Geometry check sheet. Reference: the model listing, model coordinates, mm. Round coordinates to 2 decimals unless told otherwise and drop trailing zeros. Order: outer loops, then holes, each group sorted by start corner. A loop starts at its lowest first (then second) coordinate and runs counter-clockwise, first axis right, second up. Notation, with made-up numbers: (88, 24) - (142, 24) arc R18 ccw to (142, 48) - close; hole circle Ø1 at (-16, 13.5). An arc over 180 degrees is marked (long way). Answer as CSV lines item,"result". Start each with the question number.
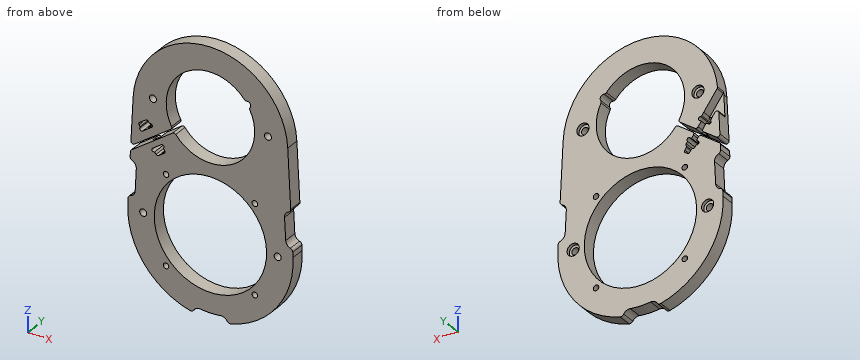
```python
from build123d import *

# Parameters (mm, degrees)
SKETCH1_R           = 40
SKETCH1_R_2         = 50.8
SKETCH1_R_3         = 2.5
BOSS_EXTRUDE1_DEPTH = 12.7
CUT_EXTRUDE1_DEPTH  = 194.127134292
CUT_EXTRUDE2_DEPTH  = 8.5
CUT_EXTRUDE3_DEPTH  = 8.5
CUT_EXTRUDE4_DEPTH  = 194.127134292
CUT_EXTRUDE5_DEPTH  = 8.5
FILLET1_R           = 2
FILLET2_R           = 2
FILLET3_R           = 1.6
FILLET4_R           = 1
SKETCH10_R          = 3.175
CUT_EXTRUDE6_DEPTH  = 194.127134292
SKETCH11_R          = 3
CUT_EXTRUDE7_DEPTH  = 194.127134292
FILLET5_R           = 2
SKETCH12_R          = 5.5
CUT_EXTRUDE8_DEPTH  = 3
CUT_EXTRUDE9_DEPTH  = 194.12713443
FILLET6_R           = 3


with BuildPart() as part:
    # Sketch1 → Boss-Extrude1 (new body)
    with BuildSketch(Plane(origin=(0, 0, 0), x_dir=(1, 0, 0), z_dir=(0, 1, 0))):
        with BuildLine():
            Line((-74.704056398, 99.012658228), (-69.910213207, 4.455696203))
            ThreePointArc((-69.910213207, 4.455696203), (0, -62), (69.910213207, 4.455696203))
            Line((69.910213207, 4.455696203), (74.704056398, 99.012658228))
            ThreePointArc((74.704056398, 99.012658228), (0, 177.6), (-74.704056398, 99.012658228))
        make_face()
        with Locations(Location((0, 0, 0), (0, 0, 270))):
            Circle(SKETCH1_R, mode=Mode.SUBTRACT)
        with Locations(Location((0, 102.8, 0), (0, 0, 270))):
            Circle(SKETCH1_R_2, mode=Mode.SUBTRACT)
        with Locations(Location((40.163665171, 142.963665171, 0), (0, 0, 270))):
            Circle(SKETCH1_R_3, mode=Mode.SUBTRACT)
        with Locations(Location((40.163665171, 62.636334829, 0), (0, 0, 270))):
            Circle(SKETCH1_R_3, mode=Mode.SUBTRACT)
        with Locations(Location((-40.163665171, 62.636334829, 0), (0, 0, 270))):
            Circle(SKETCH1_R_3, mode=Mode.SUBTRACT)
        with Locations(Location((-40.163665171, 142.963665171, 0), (0, 0, 270))):
            Circle(SKETCH1_R_3, mode=Mode.SUBTRACT)
    extrude(amount=BOSS_EXTRUDE1_DEPTH)

    # Sketch3 → Cut-Extrude1 (cut, through all)
    with BuildSketch(Plane(origin=(0, 12.7, 0), x_dir=(1, 0, 0), z_dir=(0, 1, 0))):
        Polygon((0, 0), (-72.307134802, 51.734177215), (-74.169151375, 49.131698727), (-1.862016573, -2.602478489), align=None)
    extrude(amount=-CUT_EXTRUDE1_DEPTH, mode=Mode.SUBTRACT)

    # Sketch4 → Cut-Extrude2 (cut)
    with BuildSketch(Plane(origin=(0, 12.7, 0), x_dir=(1, 0, 0), z_dir=(0, 1, 0))):
        Polygon((-55.43094311, 35.72491958), (-72.445263355, 11.944571389), (-69.985011402, 5.93106572), (-50.957933208, 32.524578595), align=None)
    extrude(amount=-CUT_EXTRUDE2_DEPTH, mode=Mode.SUBTRACT)

    # Sketch5 → Cut-Extrude3 (cut)
    with BuildSketch(Plane(origin=(0, 12.7, 0), x_dir=(1, 0, 0), z_dir=(0, 1, 0))):
        Polygon((-50.957933208, 32.524578595), (-39.203953593, 48.952724054), (-43.676963495, 52.153065038), (-55.43094311, 35.72491958), align=None)
    extrude(amount=-CUT_EXTRUDE3_DEPTH, mode=Mode.SUBTRACT)

    # Sketch6 → Cut-Extrude4 (cut, through all)
    with BuildSketch(Plane(origin=(0, 12.7, 0), x_dir=(1, 0, 0), z_dir=(0, 1, 0))):
        with BuildLine():
            Line((-61.399034012, 31.387778703), (-53.136164811, 25.475876085))
            ThreePointArc((-53.136164811, 25.475876085), (-52.765933853, 23.243628554), (-54.998181384, 22.873397596))
            Line((-54.998181384, 22.873397596), (-57.209326064, 19.782954391))
            Line((-57.209326064, 19.782954391), (-65.472195265, 25.694857009))
            Line((-65.472195265, 25.694857009), (-63.261050585, 28.785300214))
            ThreePointArc((-63.261050585, 28.785300214), (-63.631281543, 31.017547745), (-61.399034012, 31.387778703))
        make_face()
        with BuildLine():
            Line((-48.253577172, 49.279546767), (-40.446141706, 43.693497049))
            Line((-40.446141706, 43.693497049), (-42.657286386, 40.603053844))
            ThreePointArc((-42.657286386, 40.603053844), (-42.287055428, 38.370806313), (-44.519302959, 38.000575355))
            Line((-44.519302959, 38.000575355), (-52.326738425, 43.586625073))
            ThreePointArc((-52.326738425, 43.586625073), (-52.696969382, 45.818872604), (-50.464721852, 46.189103562))
            Line((-50.464721852, 46.189103562), (-48.253577172, 49.279546767))
        make_face()
    extrude(amount=-CUT_EXTRUDE4_DEPTH, mode=Mode.SUBTRACT)

    # Sketch7 → Cut-Extrude5 (cut)
    with BuildSketch(Plane(origin=(0, 12.7, 0), x_dir=(1, 0, 0), z_dir=(0, 1, 0))):
        Polygon((-57.209326064, 19.782954391), (-69.762440014, 2.237885514), (-73.208758404, 10.192307077), (-70.622080139, 18.497034605), (-65.472195265, 25.694857009), align=None)
    extrude(amount=-CUT_EXTRUDE5_DEPTH, mode=Mode.SUBTRACT)

    # Fillet1
    fillet1_edges = [part.edges().sort_by_distance(p)[0] for p in [
        (-32.530981106, 6.35, -23.275207158),
        (-34.288731446, 6.35, -20.598128455),
        (-72.100144873, 6.35, -47.65136972),
        (-72.307134802, 6.35, -51.734177215),
    ]]
    fillet(fillet1_edges, radius=FILLET1_R)

    # Fillet2
    fillet2_edges = [part.edges().sort_by_distance(p)[0] for p in [
        (-70.622080139, 8.45, -18.497034605),
        (-69.762440014, 8.45, -2.237885514),
        (-55.43094311, 8.45, -35.72491958),
        (-50.957933208, 8.45, -32.524578595),
        (-53.568926538, 8.45, -38.327398068),
        (-49.095916635, 8.45, -35.127057084),
    ]]
    fillet(fillet2_edges, radius=FILLET2_R)

    # Fillet3
    fillet3_edges = [part.edges().sort_by_distance(p)[0] for p in [
        (-57.209326064, 2.1, -19.782954391),
        (-65.472195265, 2.1, -25.694857009),
        (-48.253577172, 6.35, -49.279546767),
        (-40.446141706, 6.35, -43.693497049),
        (-39.203953593, 8.45, -48.952724054),
        (-43.676963495, 8.45, -52.153065038),
    ]]
    fillet(fillet3_edges, radius=FILLET3_R)

    # Fillet4
    # the kernel refuses this fillet: 1 mm, written as the material it takes off along each edge
    with BuildSketch(Plane(origin=(-54.998181384, 14.7, -22.873397596), x_dir=(0.9115973776641382, 0, 0.41108420188066924), z_dir=(0, -1, 0))) as fillet4_piece_1:
        with BuildLine():
            CenterArc((0.823687768, 0.980580676), FILLET4_R, 191.309932474, 67.380135052)
            Line((-0.156892908, 0.784464541), (0, 0))
            ThreePointArc((0, 0), (0.313785816, 0.031070919), (0.627571632, 0))
        make_face()
    extrude(amount=16.7, mode=Mode.SUBTRACT)
    with BuildSketch(Plane(origin=(-63.261050585, 14.7, -28.785300214), x_dir=(-0.6833651940435568, 0, -0.7300767162222146), z_dir=(0, -1, 0))) as fillet4_piece_2:
        with BuildLine():
            CenterArc((0.823687768, -0.980580676), FILLET4_R, 101.309932474, 67.380135052)
            Line((-0.156892908, -0.784464541), (0, 0))
            ThreePointArc((0, 0), (0.313785816, -0.031070919), (0.627571632, 0))
        make_face()
    extrude(amount=16.7, mode=Mode.SUBTRACT)
    with BuildSketch(Plane(origin=(-42.113354488, 15.05290288, -44.886351416), x_dir=(0.5818801789556023, 0, -0.8132745276587705), z_dir=(0, -1, 0)), Plane(origin=(-46.58636439, 4.2, -48.0866924), x_dir=(0.5818801789556058, 0, -0.813274527658768), z_dir=(0, 1, 0))) as fillet4_piece_3:
        with BuildLine():
            CenterArc((0.941161152, 1), FILLET4_R, 192.212525269, 77.787474731)
            Line((-0.036208522, 0.788461538), (-0.133945489, 0.767307692))
            ThreePointArc((-0.133945489, 0.767307692), (-0.1, 0.45), (-0.1, 0))
            Line((-0.1, 0), (0, -0.1))
            Line((0, -0.1), (0.941161152, -0.1))
            Line((0.941161152, -0.1), (0.941161152, 0))
        make_face()
    extrude(amount=10.85290288, mode=Mode.SUBTRACT)

    # Sketch10 → Cut-Extrude6 (cut, through all)
    with BuildSketch(Plane(origin=(0, 12.7, 0), x_dir=(1, 0, 0), z_dir=(0, 1, 0))):
        with Locations(Location((-52, 0, 0), (0, 0, 270))):
            Circle(SKETCH10_R)
        with Locations(Location((-60.8, 102.8, 0), (0, 0, 270))):
            Circle(SKETCH10_R)
        with Locations(Location((60.8, 102.8, 0), (0, 0, 90))):
            Circle(SKETCH10_R)
        with Locations(Location((52, 0, 0), (0, 0, 90))):
            Circle(SKETCH10_R)
    extrude(amount=-CUT_EXTRUDE6_DEPTH, mode=Mode.SUBTRACT)

    # Sketch11 → Cut-Extrude7 (cut, through all)
    with BuildSketch(Plane(origin=(0, 12.7, 0), x_dir=(1, 0, 0), z_dir=(0, 1, 0))):
        with Locations((33.397146804, -22.01432682)):
            Circle(SKETCH11_R)
    extrude(amount=-CUT_EXTRUDE7_DEPTH, mode=Mode.SUBTRACT)

    # Fillet5
    fillet5_edges = [part.edges().sort_by_distance(p)[0] for p in [
        (34.95313052, 6.35, 19.449387313),
        (31.653304138, 6.35, 24.455435739),
    ]]
    fillet(fillet5_edges, radius=FILLET5_R)

    # Sketch12 → Cut-Extrude8 (cut)
    with BuildSketch(Plane(origin=(0, 12.7, 0), x_dir=(1, 0, 0), z_dir=(0, 1, 0))):
        with Locations(Location((-60.8, 102.8, 0), (0, 0, 270))):
            Circle(SKETCH12_R)
        with Locations(Location((60.8, 102.8, 0), (0, 0, 270))):
            Circle(SKETCH12_R)
        with Locations(Location((52, 0, 0), (0, 0, 270))):
            Circle(SKETCH12_R)
        with Locations(Location((-52, 0, 0), (0, 0, 270))):
            Circle(SKETCH12_R)
    extrude(amount=-CUT_EXTRUDE8_DEPTH, mode=Mode.SUBTRACT)

    # Sketch13 → Cut-Extrude9 (cut, through all)
    with BuildSketch(Plane(origin=(0, 12.7, 0), x_dir=(1, 0, 0), z_dir=(0, 1, 0))):
        with BuildLine():
            Line((-67.031392983, 66.171925083), (-68.044051211, 86.146271714))
            ThreePointArc((-68.044051211, 86.146271714), (-74.340152668, 91.834778235), (-80.028659189, 85.538676777))
            Line((-80.028659189, 85.538676777), (-79.016000961, 65.564330147))
            ThreePointArc((-79.016000961, 65.564330147), (-72.719899504, 59.875823626), (-67.031392983, 66.171925083))
        make_face()
        with BuildLine():
            Line((67.031392983, 66.171925083), (68.044051211, 86.146271714))
            ThreePointArc((68.044051211, 86.146271714), (74.340152668, 91.834778235), (80.028659189, 85.538676777))
            Line((80.028659189, 85.538676777), (79.016000961, 65.564330147))
            ThreePointArc((79.016000961, 65.564330147), (72.719899504, 59.875823626), (67.031392983, 66.171925083))
        make_face()
        with BuildLine():
            ThreePointArc((10.777978726, 182.877931883), (0, 183.6), (-10.777978726, 182.877931883))
            ThreePointArc((-10.777978726, 182.877931883), (-15.924014851, 176.131205847), (-9.177288816, 170.985169722))
            ThreePointArc((-9.177288816, 170.985169722), (0, 171.6), (9.177288816, 170.985169722))
            ThreePointArc((9.177288816, 170.985169722), (15.924014851, 176.131205847), (10.777978726, 182.877931883))
        make_face()
    extrude(amount=-CUT_EXTRUDE9_DEPTH, mode=Mode.SUBTRACT)

    # Fillet6
    fillet6_edges = [part.edges().sort_by_distance(p)[0] for p in [
        (-74.340152668, 6.35, -91.834778235),
        (-72.719899504, 6.35, -59.875823626),
        (74.340152668, 6.35, -91.834778235),
        (72.719899504, 6.35, -59.875823626),
        (-15.887130952, 6.35, -175.893358591),
        (15.887130952, 6.35, -175.893358591),
    ]]
    fillet(fillet6_edges, radius=FILLET6_R)


solid = part.part
```
1. Thickness scan on probe 1 along X at (y, z) = (10.4, -102.8); probe 2 along Z at (x, y) = (-35.5, 7.5); probe 3 along Z at (x, y) = (33, 8.5). Record the ranges inside material, lowest first.
2. Section check C-C on x = 60.8. Record the boundary of the cut face in (y, z) (3 decimals).
3. Section check A-A on x = 0. Record the boundary of the cut face in (y, z), plus the area to 3 significant figures.
4. Section check B-B on z = -102.8. Record the boundary of the cut face in (x, y) (3 decimals), plus the area to 3 significant figures.
5. Go/stop test with flat-tipped pins: pin 1 Ø5.5 at (x, z) = (62.5, -103) entering from +Y; pin 2 Ø1 at (x, y) = (44.5, 11) entering from -Z; pin 3 Ø3 at (x, y) = (-28, 3.5) entering from -Z. Record where each tip stops, or that it passes through.
6. Section check D-D on y = 7.5. Count the separate pieces of the cut face and the enclosed holes in it, plus the area to 3 significant figures.
Numbers:
1,probe 1,"x = -74.8 to -66.3, -55.3 to -50.8, 50.8 to 55.3, 66.3 to 74.8"
1,probe 2,"z = -168.64 to -139.14, -66.46 to -25.4, -21.43 to -18.43, 18.43 to 52.33"
1,probe 3,"z = -169.93 to -141.42, -64.18 to -22.61, 24.99 to 53.73"
2,outline,"(0, -146.371) - (12.7, -146.371) - (12.7, -108.3) - (9.7, -108.3) - (9.7, -105.975) - (0, -105.975) - close; (0, -99.625) - (9.7, -99.625) - (9.7, -97.3) - (12.7, -97.3) - (12.7, 26.689) - (0, 26.689) - close"
3,outline,"(0, -171.6) - (12.7, -171.6) - (12.7, -153.6) - (0, -153.6) - close; (0, -52) - (12.7, -52) - (12.7, -40) - (0, -40) - close; (0, 40) - (12.7, 40) - (12.7, 62) - (0, 62) - close"
3,area,"660 mm2"
4,outline,"(-74.8, 0) - (-63.975, 0) - (-63.975, 9.7) - (-66.3, 9.7) - (-66.3, 12.7) - (-74.8, 12.7) - close; (-57.625, 0) - (-50.8, 0) - (-50.8, 12.7) - (-55.3, 12.7) - (-55.3, 9.7) - (-57.625, 9.7) - close; (50.8, 0) - (57.625, 0) - (57.625, 9.7) - (55.3, 9.7) - (55.3, 12.7) - (50.8, 12.7) - close; (63.975, 0) - (74.8, 0) - (74.8, 12.7) - (66.3, 12.7) - (66.3, 9.7) - (63.975, 9.7) - close"
4,area,"420 mm2"
5,pin 1,"stops at y = 9.7"
5,pin 2,"stops at z = -163.29"
5,pin 3,"stops at z = -172.75"
6,separate pieces,"2"
6,enclosed holes,"9"
6,area,"15,800 mm2"
